Could you check a few things on this model? Use its own coordinates, in mm. Face numbers are marked on the shaded views. A direction names the side the tool comes from. Coordinates: 2 decimals unless noted, no trailing zeros. Order: outer loops, then holes, each group sorted by start corner. A loop starts at its lowest first (then second) coordinate and runs counter-clockwise, first axis right, second up. Notation, with made-up numbers: (-25.75, 61.25) - (-20.75, 61.25) arc R13 ccw to (-20.75, 79.25) - close; hole circle Ø6 at (83, 84). An arc over 180 degrees is marked (long way). Answer as a JSON object with one key per item and string values. Group by question number.
(1) Which directions (+Z, -Z, +X, -X, +Y, -Y) give clear straight access to the entire face, cutting with the end or side of a thin tool? Please do the marked faces 1 and 2.
(2) Please list where these lines run through material, in increasing order: probe 1 along Z at (x, y) = (2, 6); probe 2 along Z at (x, y) = (-7, -8.75); probe 3 along X at (y, z) = (-1.25, 8).
(3) Imagine slicing it at C-C, the plane z = 25. Write out the boundary of the cut face in (x, y).
(4) Will these pins go through, and if not, where does the flat tip stop? P1, Ø1.5, axis at x = -9, y = 3.5, coming from the +Z side; P2, Ø1.5, axis at x = -6.17, z = 8.76, coming from the -Y side; P3, Ø6, axis at x = 5.5, z = 23, coming from the +Y side.
(5) Imagine slicing it at D-D, the plane y = 6.5. Write out the boundary of the cut face in (x, z).
(6) Imagine slicing it at A-A, the plane y = 0. Write out the boundary of the cut face in (x, z).
(7) Imagine slicing it at B-B, the plane x = 0. Write out the boundary of the cut face in (y, z), and give its area (3 significant figures).
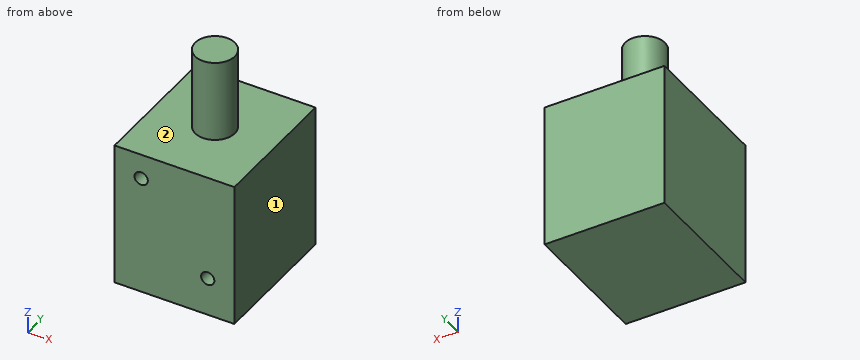
from build123d import *

# Parameters (mm, degrees)
F0_W     = 22.225
F0_H     = 26.8732
F1_DEPTH = 12.6365
F2_R     = 3.683
F3_DEPTH = 15.113
F5_D     = 2.4638
F5_DEPTH = 14.2
F5_TIP   = 0.7402001966


with BuildPart() as f1:
    # F0 (on Front) → F1 (new body, symmetric)
    with BuildSketch(Plane.XZ):
        Rectangle(F0_W, F0_H)
    extrude(amount=F1_DEPTH, both=True)

    # F2 (on face) → F3 (join)
    with BuildSketch(Plane.XY.offset(13.4366)):
        Circle(F2_R)
    extrude(amount=F3_DEPTH)

    # F5
    with Locations(Plane.XZ.offset(12.6365)):
        with Locations((-6.1722, 8.763), (6.1722, -6.3246)):
            Hole(F5_D / 2, depth=F5_DEPTH)
            with Locations((0, 0, -(F5_DEPTH + F5_TIP / 2))):  # 118° drill point
                Cone(0, F5_D / 2, F5_TIP, mode=Mode.SUBTRACT)


solid = f1.part
Result set:
{
 "1": {"face 1": "+Z, -Z, +X, +Y, -Y", "face 2": "+Z"},
 "2": {"probe 1": "z = -13.44 to 13.44", "probe 2": "z = -13.44 to 7.85, 9.68 to 13.44", "probe 3": "x = -11.11 to -7.14, -5.21 to 11.11"},
 "3": {"outline": "circle Ø7.37 at (0, 0)"},
 "4": {"P1": "stops at z = 13.44", "P2": "stops at y = 1.85", "P3": "stops at y = 2.7"},
 "5": {"outline": "(-11.11, -13.44) - (11.11, -13.44) - (11.11, 13.44) - (-11.11, 13.44) - close"},
 "6": {"outline": "(-11.11, -13.44) - (11.11, -13.44) - (11.11, 13.44) - (3.68, 13.44) - (3.68, 28.55) - (-3.68, 28.55) - (-3.68, 13.44) - (-11.11, 13.44) - close; hole circle Ø2.46 at (-6.17, 8.76); hole circle Ø2.46 at (6.17, -6.32)"},
 "7": {"outline": "(-12.64, -13.44) - (12.64, -13.44) - (12.64, 13.44) - (3.68, 13.44) - (3.68, 28.55) - (-3.68, 28.55) - (-3.68, 13.44) - (-12.64, 13.44) - close", "area": "790 mm^2"}
}
